The figure shows three views and two pictorial views of one solid part (mm, origin at its lowest corner). Answer the questions. Round coordinates to 2 decimals unless told otherwise and drop trailing zeros. Order: outer loops, then holes, each group sorted by start corner. A loop starts at its lowest first (then second) coordinate and runs counter-clockwise, first axis right, second up. Notation, with made-up numbers: (37, 10) -> (50, 10) arc R28 ccw to (50, 49) -> close; hole circle Ø10 at (-11.5, 30). An arc over 180 degrees is marked (long way). Answer in a Markdown table with one row per item. Add a question column.
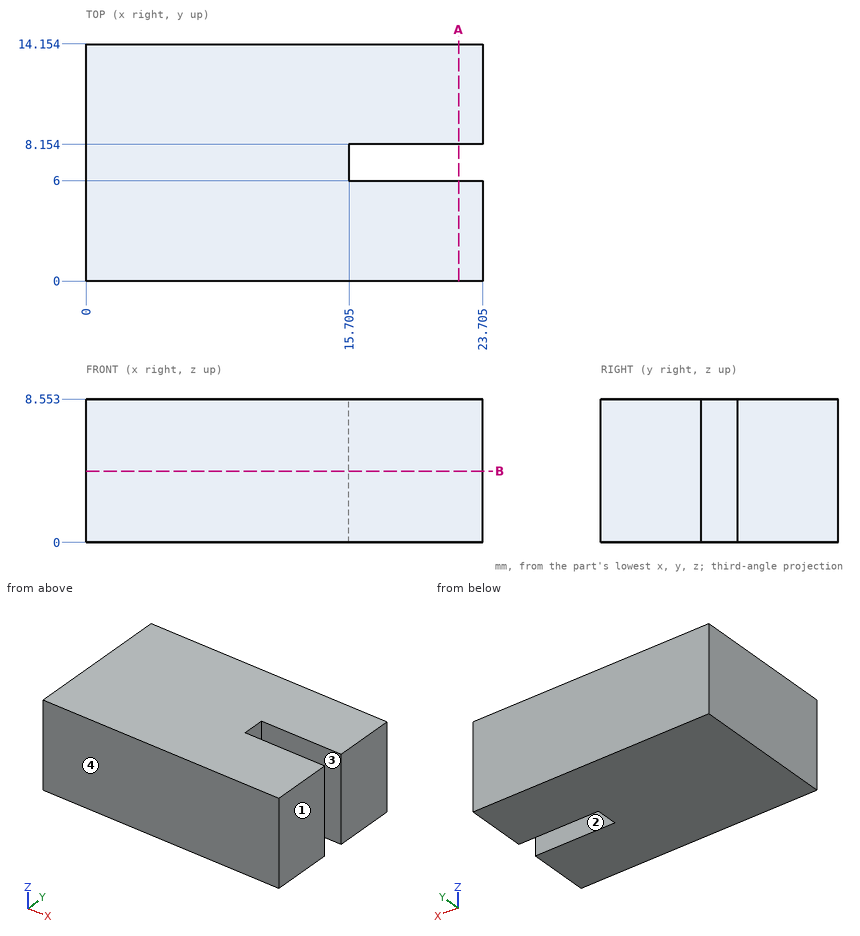
1. The mould has two halves that part along Y. Classify the marked faces 1, 2, 3 and 4: released by +Y, released by -Y, zero draft, split by the parting line, or undercut.
2. The part is cut by section B-B (z = 4.25). Give the vertices of the cut face in (x, y) (1 decimal).
3. The part is cut by section A-A (x = 22.25). Give the vertices of the cut face in (y, z).
4. Straight lines are drawn through the part: line 1 along Y through (x, z) = (19, 4); line 2 along X through (y, z) = (7.5, 6) (1 decimal). For each, find the intervals that lie inside material, in ascending order.
Report:
| question | item | result |
|---|---|---|
| 1 | face 1 | zero draft |
| 1 | face 2 | undercut |
| 1 | face 3 | undercut |
| 1 | face 4 | released by -Y |
| 2 | outline | (0, 0) -> (23.7, 0) -> (23.7, 6) -> (15.7, 6) -> (15.7, 8.2) -> (23.7, 8.2) -> (23.7, 14.2) -> (0, 14.2) -> close |
| 3 | outline | (0, 0) -> (6, 0) -> (6, 8.55) -> (0, 8.55) -> close; (8.15, 0) -> (14.15, 0) -> (14.15, 8.55) -> (8.15, 8.55) -> close |
| 4 | line 1 | y = 0 to 6, 8.15 to 14.15 |
| 4 | line 2 | x = 0 to 15.7 |
